```python
from build123d import *

# Parameters (mm, degrees)
BOSS_EXTRUDE1_DEPTH = 275
SKETCH2_R           = 4
CUT_EXTRUDE1_DEPTH  = 2.5875
CUT_EXTRUDE2_START  = -2.5875
SKETCH3_R           = 3
CUT_EXTRUDE2_DEPTH  = 27.4


with BuildPart() as part:
    # Sketch1 → Boss-Extrude1 (new body, symmetric)
    with BuildSketch(Plane.XY):
        Polygon((0, 0), (0, 25.4), (1.5875, 25.4), (1.5875, 1.5875), (25.4, 1.5875), (25.4, 0), align=None)
    extrude(amount=BOSS_EXTRUDE1_DEPTH, both=True)

    # Sketch2 → Cut-Extrude1 (cut, through all)
    with BuildSketch(Plane(origin=(1.5875, 0, 0), x_dir=(0, 0, -1), z_dir=(1, 0, 0))):
        with Locations((265, 12.7)):
            Circle(SKETCH2_R)
        with Locations((206.2, 12.7)):
            Circle(SKETCH2_R)
        with Locations((147.4, 12.7)):
            Circle(SKETCH2_R)
        with Locations((88.6, 12.7)):
            Circle(SKETCH2_R)
        with Locations((29.8, 12.7)):
            Circle(SKETCH2_R)
        with Locations((-29, 12.7)):
            Circle(SKETCH2_R)
        with Locations((-87.8, 12.7)):
            Circle(SKETCH2_R)
        with Locations((-146.6, 12.7)):
            Circle(SKETCH2_R)
        with Locations((-205.4, 12.7)):
            Circle(SKETCH2_R)
        with Locations((-264.2, 12.7)):
            Circle(SKETCH2_R)
    extrude(amount=-CUT_EXTRUDE1_DEPTH, mode=Mode.SUBTRACT)

    # Sketch3 → Cut-Extrude2 (cut)
    with BuildSketch(Plane(origin=(0, 1.5875, 0), x_dir=(1, 0, 0), z_dir=(0, 1, 0)).offset(CUT_EXTRUDE2_START)):
        with Locations((13, 265)):
            Circle(SKETCH3_R)
    cut_extrude2 = extrude(amount=CUT_EXTRUDE2_DEPTH, mode=Mode.SUBTRACT)

    # Mirror1: Cut-Extrude2 across plane
    add(cut_extrude2.mirror(Plane.XY), mode=Mode.SUBTRACT)


solid = part.part
```
For this review, take the finished solid that the model builds, in its own axes (mm). A direction names the side the tool comes from. Round coordinates to 2 decimals unless told otherwise and drop trailing zeros. Write each loop counter-clockwise with the first axis right and the second up, starting at its lowest first coordinate (ties: lowest second). Pieces come first, ordered by that corner, then holes. Notation, with made-up numbers: (31.25, 86) -> (49.25, 86) arc R14 ccw to (49.25, 94) -> close; hole circle Ø4 at (75.5, -10.5). An arc over 180 degrees is marked (long way). Use one line per item in the form item = value.
1) Tool access review of faces 1 (the flat face through (7, 1, -275)), 2 (the flat face through (1.588, 14, 4)): name each direction out of +Z, -Z, +X, -X, +Y, -Y from which nothing blocks a thin tool from reaching the whole face with its end or side.
Found:
face_1 = -Z, +X, -X, +Y, -Y
face_2 = +Z, -Z, +X, +Y
2) Clearance check with flat-ended pins moving along their axes: pin 1 (12 mm diameter, centred on y = 12, z = -91.5, fed in from +X); pin 2 (6.5 mm diameter, centred on y = 12.7, z = 87.8, fed in from -X); pin 3 (7 mm diameter, centred on x = 14, z = -0.5, fed in from +Y). State where each tip first meets the part, or that it passes through.
Found:
pin_1 = 1.59
pin_2 = through
pin_3 = 1.59
3) Take a section at A-A, the plane z = -215. Write out the cut boundary in (x, y), and give its area (3 significant figures).
Found:
outline = (0, 0) -> (25.4, 0) -> (25.4, 1.59) -> (1.59, 1.59) -> (1.59, 25.4) -> (0, 25.4) -> close
area = 78.1 mm2
4) To check wall thickness, follow L1, parallel to Z at x = 13, y = 0.4; L2, parallel to X at y = 1.1, z = -265; L3, parallel to Y at x = 10.5, z = -166.5. State the ranges of each line that lie inside material, in increasing order. Write a range as from..to.
Found:
L1 = -275..-268, -262..262, 268..275
L2 = 0..10, 16..25.4
L3 = 0..1.59
5) Take a section at B-B, the plane y = 12.7. Count the separate pieces of the cut face and the enclosed holes in it, and give its area (3 significant figures).
Found:
separate_pieces = 11
enclosed_holes = 0
area = 746 mm2
